CAD build for the part. Positions are in the model's coordinates, mm. A direction names the side the tool comes from. Round coordinates to 2 decimals unless told otherwise and drop trailing zeros. Loops run counter-clockwise (first coordinate to the right, second up) from the corner with the lowest first, then second, coordinate; pieces in that order, holes last.
from build123d import *

# Parameters (mm, degrees)
F0_R     = 38.1
F0_R_2   = 3.175
F1_DEPTH = 3.302
F2_DEPTH = 101.6
F3_R     = 38.08114
F3_R_2   = 3.175
F4_DEPTH = 3.302
F6_R     = 1.397
F6_R_2   = 6.35
F7_DEPTH = 136.906


with BuildPart() as f1:
    # F0 (on Top) → F1 (new body)
    with BuildSketch(Plane.XY):
        Circle(F0_R)
        Polygon((-19.714349, -27.997382), (-20.965572, -27.06588), (-10.624112, -16.024547), (-9.259141, -17.040731), align=None, mode=Mode.SUBTRACT)
        Polygon((-32.427083, -10.999691), (-32.888933, -9.50974), (-18.027077, -6.684488), (-17.52324, -8.309888), align=None, mode=Mode.SUBTRACT)
        Polygon((0.573601, -34.237113), (-0.986216, -34.221988), (0.861155, -19.207194), (2.562772, -19.223693), align=None, mode=Mode.SUBTRACT)
        Polygon((20.641144, -27.321275), (19.372093, -28.228339), (12.015524, -15.009499), (13.399943, -14.019975), align=None, mode=Mode.SUBTRACT)
        Polygon((32.777353, -9.907271), (32.286698, -11.387985), (18.552942, -5.044423), (19.088202, -3.429099), align=None, mode=Mode.SUBTRACT)
        Polygon((-32.679751, 10.224618), (-32.174761, 11.700505), (-18.503159, 5.224077), (-19.054056, 3.614019), align=None, mode=Mode.SUBTRACT)
        Polygon((-20.375264, 27.52013), (-19.097477, 28.414846), (-11.869425, 15.125297), (-13.263374, 14.149244), align=None, mode=Mode.SUBTRACT)
        Polygon((-2.749047, 19.197941), (-0.905541, 34.229942), (0.654349, 34.229942), (-1.04735, 19.197941), align=None, mode=Mode.SUBTRACT)
        Circle(F0_R_2, mode=Mode.SUBTRACT)
        Polygon((32.318904, 11.31359), (32.795179, 9.828188), (17.961416, 6.858967), (17.441843, 8.479405), align=None, mode=Mode.SUBTRACT)
        Polygon((19.441956, 28.187218), (20.702153, 27.267892), (10.468237, 16.126807), (9.093476, 17.129707), align=None, mode=Mode.SUBTRACT)
    extrude(amount=F1_DEPTH)

    # F0 (on Top) → F2 (join)
    with BuildSketch(Plane.XY):
        Polygon((-18.503159, 5.224077), (-32.174761, 11.700505), (-32.679751, 10.224618), (-19.054056, 3.614019), align=None)
        Polygon((-18.027077, -6.684488), (-32.888933, -9.50974), (-32.427083, -10.999691), (-17.52324, -8.309888), align=None)
        Polygon((-10.624112, -16.024547), (-20.965572, -27.06588), (-19.714349, -27.997382), (-9.259141, -17.040731), align=None)
        Polygon((0.861155, -19.207194), (-0.986216, -34.221988), (0.573601, -34.237113), (2.562772, -19.223693), align=None)
        Polygon((12.015524, -15.009499), (19.372093, -28.228339), (20.641144, -27.321275), (13.399943, -14.019975), align=None)
        Polygon((18.552942, -5.044423), (32.286698, -11.387985), (32.777353, -9.907271), (19.088202, -3.429099), align=None)
        Polygon((17.961416, 6.858967), (32.795179, 9.828188), (32.318904, 11.31359), (17.441843, 8.479405), align=None)
        Polygon((10.468237, 16.126807), (20.702153, 27.267892), (19.441956, 28.187218), (9.093476, 17.129707), align=None)
        Polygon((0.654349, 34.229942), (-0.905541, 34.229942), (-2.749047, 19.197941), (-1.04735, 19.197941), align=None)
        Polygon((-11.869425, 15.125297), (-19.097477, 28.414846), (-20.375264, 27.52013), (-13.263374, 14.149244), align=None)
    extrude(amount=F2_DEPTH)

    # F3 (on face) → F4 (join)
    with BuildSketch(Plane.XY.offset(101.6)):
        Circle(F3_R)
        Circle(F3_R_2, mode=Mode.SUBTRACT)
    extrude(amount=F4_DEPTH)

    # F6 (on face) → F7 (cut)
    with BuildSketch(Plane.XY):
        with Locations((6.985, -6.985001)):
            Circle(F6_R)
        with Locations((-6.985, -6.985001)):
            Circle(F6_R)
        with Locations((-6.985, 6.985001)):
            Circle(F6_R)
        with Locations((6.985, 6.985001)):
            Circle(F6_R)
        Circle(F6_R_2)
    extrude(amount=F7_DEPTH, mode=Mode.SUBTRACT)


solid = f1.part
Item 1: 3-axis set-ups, long thin cutter, end or side, ignore diameter. For faces 1 (the flat face through (-1.814, 26.819, 51.763)), 2 (the flat face through (-25.962, 6.966, 51.763)), 3 (the flat face through (25.27, 8.32, 51.76)): which of +Z, -Z, +X, -X, +Y, -Y reach the whole face in a straight line?
Verdict:
face 1: +Y
face 2: -X
face 3: +X
Item 2: Mould opens along X. For faces 4 (the flat face through (8, 1, 0)), 5 (the flat face through (15.514, 21.619, 51.763)), 6 (the flat face through (15.642, -21.526, 51.763)), 7 (the flat face through (-0.21, 26.61, 51.76)) say: released by +X, released by -X, zero draft, split by the parting line, or undercut.
Verdict:
face 4: zero draft
face 5: released by +X
face 6: undercut
face 7: undercut
Item 3: Flat gauge pins, fed straight in: P1, Ø8, axis at x = -11, z = 80, coming from the +Y side; P2, Ø1.7, axis at x = -0.5, z = 66.5, coming from the +Y side; P3, Ø2, axis at x = -6.985, y = 6.985, coming from the -Z side; P4, Ø5, axis at y = -21.5, z = 36, coming from the +X side. Where does each tip first touch, or does it go through?
Verdict:
P1: stops at y = 20.88
P2: stops at y = 34.23
P3: passes through
P4: stops at x = 18.83
Item 4: Wall check: L1, parallel to Z at x = 10, y = 11; L2, parallel to Y at x = 0, z = 102; L3, parallel to X at y = 25.5, z = 91.5. Give the ranges that are in metal, low to high.
Verdict:
L1: z = 0 to 3.3, 101.6 to 104.9
L2: y = -38.08 to -6.35, 6.35 to 38.08
L3: x = -19.3 to -17.51, -1.98 to -0.33, 16.93 to 19.08
Item 5: Cut at A-A (y = 0). List the corners of the cut face in (x, z).
Verdict:
outline: (-38.1, 0) - (-6.35, 0) - (-6.35, 3.3) - (-38.1, 3.3) - close; (-38.08, 101.6) - (-6.35, 101.6) - (-6.35, 104.9) - (-38.08, 104.9) - close; (6.35, 0) - (38.1, 0) - (38.1, 3.3) - (6.35, 3.3) - close; (6.35, 101.6) - (38.08, 101.6) - (38.08, 104.9) - (6.35, 104.9) - close
Item 6: Cut at C-C (z = 43). State how many separate pieces and enclosed holes the cut face has, plus the area to 3 significant figures.
Verdict:
separate pieces: 10
enclosed holes: 0
area: 245 mm2
Item 7: Cut at B-B (x = -23.5). List the corners of the cut face in (y, z).
Verdict:
outline: (-29.99, 0) - (29.99, 0) - (29.99, 3.3) - (7.59, 3.3) - (7.59, 101.6) - (29.97, 101.6) - (29.97, 104.9) - (-29.97, 104.9) - (-29.97, 101.6) - (-9.39, 101.6) - (-9.39, 3.3) - (-29.99, 3.3) - close; hole (-7.72, 3.3) - (5.77, 3.3) - (5.77, 101.6) - (-7.72, 101.6) - close
Item 8: Cut at D-D (y = -24.5). List the corners of the cut face in (x, z).
Verdict:
outline: (-29.18, 0) - (29.18, 0) - (29.18, 3.3) - (19.11, 3.3) - (19.11, 101.6) - (29.15, 101.6) - (29.15, 104.9) - (-29.15, 104.9) - (-29.15, 101.6) - (-18.56, 101.6) - (-18.56, 3.3) - (-29.18, 3.3) - close; hole (-16.38, 3.3) - (0.21, 3.3) - (0.21, 101.6) - (-16.38, 101.6) - close; hole (1.86, 3.3) - (17.3, 3.3) - (17.3, 101.6) - (1.86, 101.6) - close
